from build123d import *

# Parameters (mm, degrees)
SKETCH1_W               = 8
SKETCH1_H               = 8
BOSS_EXTRUDE1_DEPTH     = 3
CUT_EXTRUDE1_DEPTH      = 12.704699911
CUT_EXTRUDE1_DEPTH_BACK = 12.704699911
CUT_EXTRUDE2_DEPTH      = 11
SKETCH4_R               = 1.75
CUT_EXTRUDE3_DEPTH      = 0.4
SKETCH5_W               = 8
SKETCH5_H               = 1
BOSS_EXTRUDE2_DEPTH     = 2
FILLET1_R               = 4
CUT_EXTRUDE4_DEPTH      = 0.4
CUT_EXTRUDE5_DEPTH      = 0.5


with BuildPart() as part:
    # Sketch1 → Boss-Extrude1 (new body)
    with BuildSketch(Plane(origin=(0, 0, 0), x_dir=(1, 0, 0), z_dir=(0, 1, 0))):
        with Locations((4, 4)):
            Rectangle(SKETCH1_W, SKETCH1_H)
    extrude(amount=BOSS_EXTRUDE1_DEPTH)

    # Sketch2 → Cut-Extrude1 (cut, two sides: drawn at the far end of the back side and taken through both)
    with BuildSketch(Plane.XY.offset(-CUT_EXTRUDE1_DEPTH_BACK)):
        Polygon((0, 0), (0.6, 3), (0, 3), align=None)
        Polygon((8, 0), (7.4, 3), (8, 3), align=None)
    extrude(amount=CUT_EXTRUDE1_DEPTH + CUT_EXTRUDE1_DEPTH_BACK, mode=Mode.SUBTRACT)

    # Sketch3 → Cut-Extrude2 (cut)
    with BuildSketch(Plane(origin=(0, 0, 0), x_dir=(0, 0, -1), z_dir=(1, 0, 0))):
        Polygon((0, 0), (0.6, 3), (0, 3), align=None)
        Polygon((8, 3), (7.4, 3), (8, 0), align=None)
    extrude(amount=CUT_EXTRUDE2_DEPTH, mode=Mode.SUBTRACT)

    # Sketch4 → Cut-Extrude3 (cut)
    with BuildSketch(Plane.XZ):
        with Locations(Location((4, -3.75, 0), (0, 0, 270))):
            Circle(SKETCH4_R)
    extrude(amount=-CUT_EXTRUDE3_DEPTH, mode=Mode.SUBTRACT)

    # Sketch5 → Boss-Extrude2 (add)
    with BuildSketch(Plane.XZ):
        with Locations((4, -7.5)):
            Rectangle(SKETCH5_W, SKETCH5_H)
    extrude(amount=BOSS_EXTRUDE2_DEPTH)

    # Fillet1
    # the kernel refuses this fillet: 4 mm, written as the material it takes off along each edge
    with BuildSketch(Plane(origin=(8, -2, -16.660254038), x_dir=(0, 1, 0), z_dir=(0, 0, 1)), Plane(origin=(0, -2, 1.660254038), x_dir=(0, 1, 0), z_dir=(0, 0, -1))) as fillet1_piece_1:
        with BuildLine():
            CenterArc((4, 3.464101615), FILLET1_R, 180, 60)
            Line((0, 3.464101615), (-0.08, 3.464101615))
            Line((-0.08, 3.464101615), (-0.08, 0))
            Line((-0.08, 0), (0, -0.08))
            ThreePointArc((0, -0.08), (1, -0.08), (1.96, -0.069282032))
            Line((1.96, -0.069282032), (2, 0))
        make_face()
    extrude(amount=18.320508076, mode=Mode.SUBTRACT)

    # Sketch6 → Cut-Extrude4 (cut)
    with BuildSketch(Plane(origin=(0, 3, 0), x_dir=(1, 0, 0), z_dir=(0, 1, 0))):
        with BuildLine():
            Line((2.413140262, 5.995145478), (3.182371031, 5.995145478))
            Line((3.182371031, 5.995145478), (3.182371031, 3.824472401))
            add(Edge.make_bspline(
                [(3.182371031, 3.824472401), (3.182664695, 3.783339968), (3.183225327, 3.704814249), (3.183611242, 3.59262518), (3.18574694, 3.491896749), (3.190378411, 3.402466647), (3.193557117, 3.32438048), (3.199459629, 3.257623918), (3.205347836, 3.202222959), (3.211072588, 3.16927001), (3.213621031, 3.154600607)],
                knots=[0, 0, 0, 0, 1.470600056, 2.807515117, 4.011048972, 5.072079398, 6.00911328, 6.804506435, 7.467811572, 8, 8, 8, 8], degree=3))
            add(Edge.make_bspline(
                [(3.213621031, 3.154600607), (3.224127628, 3.115054038), (3.244816443, 3.03718185), (3.301842427, 2.930732637), (3.377172946, 2.83690436), (3.454012852, 2.769989694), (3.523520467, 2.722632459), (3.582561491, 2.693810163), (3.645203631, 2.667536787), (3.712771176, 2.647377448), (3.784538951, 2.629737301), (3.861373833, 2.619537644), (3.942627383, 2.611709661), (3.998321517, 2.610930314), (4.026922313, 2.610530094)],
                knots=[0, 0, 0, 0, 1.376921055, 2.711331395, 4.038631339, 5.418057255, 6.132954575, 6.870556231, 7.630397752, 8.422890386, 9.247036838, 10.121396817, 11.035274583, 12, 12, 12, 12], degree=3))
            add(Edge.make_bspline(
                [(4.026922313, 2.610530094), (4.055777389, 2.611053435), (4.111957634, 2.612072369), (4.193372399, 2.618140476), (4.269330983, 2.629588903), (4.339786919, 2.644600001), (4.40511233, 2.663571514), (4.464786061, 2.687591678), (4.518714075, 2.716497769), (4.582078678, 2.760066391), (4.650258908, 2.821527538), (4.715873674, 2.905091818), (4.762833649, 2.997337694), (4.784859868, 3.081565077), (4.796180605, 3.154949811), (4.803077806, 3.219164001), (4.809385646, 3.291832182), (4.815113647, 3.372755319), (4.819030865, 3.461994153), (4.821149619, 3.559774375), (4.82281709, 3.666080391), (4.823198873, 3.739802878), (4.823396672, 3.777998042)],
                knots=[0, 0, 0, 0, 1.036876239, 2.018776863, 2.930845756, 3.794842666, 4.605604932, 5.371924355, 6.101864688, 6.799283669, 8.1310906, 9.382718023, 10.597336334, 11.822035891, 12.492591141, 13.265194674, 14.141890321, 15.11351293, 16.179860579, 17.351049011, 18.627594861, 20, 20, 20, 20], degree=3))
            Line((4.823396672, 3.777998042), (4.823396672, 5.995145478))
            Line((4.823396672, 5.995145478), (5.592627441, 5.995145478))
            Line((5.592627441, 5.995145478), (5.592627441, 3.902998042))
            add(Edge.make_bspline(
                [(5.592627441, 3.902998042), (5.592528847, 3.845305157), (5.592339402, 3.734449864), (5.589381475, 3.574956755), (5.583094941, 3.428628514), (5.577830511, 3.295214312), (5.567675642, 3.175054503), (5.557043529, 3.068074376), (5.543346947, 2.974292627), (5.523815493, 2.867696041), (5.490991615, 2.748101531), (5.438090809, 2.615994056), (5.370481989, 2.495804532), (5.288434562, 2.387071806), (5.192421188, 2.289363714), (5.081004269, 2.203064381), (4.955329501, 2.127124651), (4.84016309, 2.072443299), (4.739752735, 2.035622669), (4.65797018, 2.010704116), (4.570444093, 1.989952175), (4.477277128, 1.973483664), (4.378429252, 1.959598273), (4.273864574, 1.950325107), (4.163741291, 1.944537997), (4.088628699, 1.944091898), (4.050159493, 1.943863427)],
                knots=[0, 0, 0, 0, 1.415574045, 2.719986624, 3.913607924, 5.00929969, 5.995467356, 6.871900228, 7.64671288, 8.320227872, 9.530145585, 10.682614022, 11.803571353, 12.90325401, 14.015460715, 15.154679255, 16.351678057, 17.612271512, 18.275764165, 18.974412946, 19.708786676, 20.481351116, 21.295095879, 22.157200529, 23.056203067, 24, 24, 24, 24], degree=3))
            add(Edge.make_bspline(
                [(4.050159493, 1.943863427), (4.00394899, 1.944454117), (3.914432357, 1.945598373), (3.784491522, 1.950702797), (3.663419731, 1.961238523), (3.550836598, 1.975478544), (3.446788608, 1.993784557), (3.351012543, 2.015669281), (3.264273035, 2.043328483), (3.160959321, 2.082832512), (3.045798952, 2.143260432), (2.920442018, 2.223870786), (2.810400187, 2.314853884), (2.716640343, 2.415320705), (2.638260762, 2.521740618), (2.574552012, 2.631810814), (2.523497916, 2.743696672), (2.502164616, 2.821459533), (2.491665903, 2.859728812)],
                knots=[0, 0, 0, 0, 1.128613534, 2.186292659, 3.174878439, 4.095586888, 4.95671962, 5.754129884, 6.492676435, 7.178284149, 8.453103036, 9.659838108, 10.813193309, 11.929983019, 13.007587775, 14.033493319, 15.032227051, 16, 16, 16, 16], degree=3))
            add(Edge.make_bspline(
                [(2.491665903, 2.859728812), (2.48524032, 2.889857793), (2.471705989, 2.953319061), (2.456334745, 3.054210037), (2.442311642, 3.165307899), (2.432733679, 3.286744058), (2.423654648, 3.418133217), (2.417136225, 3.559723113), (2.414455843, 3.711481594), (2.413587623, 3.816192051), (2.413140262, 3.870145478)],
                knots=[0, 0, 0, 0, 0.728071598, 1.533551606, 2.411422299, 3.374601532, 4.412367648, 5.524718474, 6.72457895, 8, 8, 8, 8], degree=3))
            Line((2.413140262, 3.870145478), (2.413140262, 5.995145478))
        make_face()
    extrude(amount=-CUT_EXTRUDE4_DEPTH, mode=Mode.SUBTRACT)

    # Sketch7 → Cut-Extrude5 (cut)
    with BuildSketch(Plane(origin=(0, 3, 0), x_dir=(1, 0, 0), z_dir=(0, 1, 0))):
        with BuildLine():
            Line((5.850386773, 2.400368579), (5.850386773, 2.746522425))
            Line((5.850386773, 2.746522425), (7.02730985, 2.746522425))
            Line((7.02730985, 2.746522425), (7.02730985, 2.492676271))
            add(Edge.make_bspline(
                [(7.02730985, 2.492676271), (7.015032321, 2.480184286), (6.989793248, 2.454504354), (6.953640746, 2.41247659), (6.916952595, 2.366869092), (6.880495981, 2.317067299), (6.84313767, 2.263857918), (6.806519427, 2.206220957), (6.769380335, 2.144904141), (6.719379376, 2.058171383), (6.660934493, 1.944871602), (6.599102899, 1.804034186), (6.546425212, 1.658871525), (6.510353845, 1.535182236), (6.485981829, 1.436045461), (6.470058334, 1.363554301), (6.45665413, 1.293103137), (6.44574982, 1.224568153), (6.437611625, 1.157918082), (6.431181064, 1.093384645), (6.428008496, 1.030810475), (6.427540351, 0.989794441), (6.42730985, 0.969599348)],
                knots=[0, 0, 0, 0, 0.628545797, 1.29210959, 1.98878689, 2.729126096, 3.507039704, 4.322017351, 5.179550397, 6.080149501, 7.915136253, 9.752312618, 11.597470118, 13.454141581, 14.373891568, 15.261584755, 16.117868869, 16.947726723, 17.752002974, 18.527724242, 19.275094557, 20, 20, 20, 20], degree=3))
            Line((6.42730985, 0.969599348), (6.081156004, 0.969599348))
            add(Edge.make_bspline(
                [(6.081156004, 0.969599348), (6.082313464, 1.000264514), (6.084641243, 1.061935513), (6.093350513, 1.15450167), (6.107029358, 1.247412503), (6.124019401, 1.340882746), (6.146450494, 1.434684851), (6.172051243, 1.529166286), (6.203062702, 1.623822431), (6.237825714, 1.718472296), (6.276202253, 1.812217257), (6.31802728, 1.903894573), (6.363192674, 1.992932291), (6.411111069, 2.079643245), (6.462339924, 2.16374848), (6.516917811, 2.245156666), (6.574070556, 2.324456683), (6.614935451, 2.375068877), (6.635362734, 2.400368579)],
                knots=[0, 0, 0, 0, 0.943249748, 1.896978291, 2.856365892, 3.829648507, 4.816416106, 5.820376826, 6.838120354, 7.877341886, 8.919613352, 9.951365796, 10.974227495, 11.988073359, 12.996274698, 14.000568529, 15.000536908, 16, 16, 16, 16], degree=3))
            Line((6.635362734, 2.400368579), (5.850386773, 2.400368579))
        make_face()
    extrude(amount=-CUT_EXTRUDE5_DEPTH, mode=Mode.SUBTRACT)


solid = part.part
Geometry: final body of the model. Coordinates: model frame, mm. A direction names the side the tool comes from. Coordinates: 2 decimals unless noted, no trailing zeros. Write each loop counter-clockwise with the first axis right and the second up, starting at its lowest first coordinate (ties: lowest second). Pieces come first, ordered by that corner, then holes. Notation, with made-up numbers: (36, 0) - (45, 0) arc R21 ccw to (45, 37) - close; hole circle Ø7 at (-28.75, 49.5). An arc over 180 degrees is marked (long way). Return JSON: item names as keys, results as strings.
Item 1: Line query: L1, parallel to Y at x = 1.75, z = -4.5; L2, parallel to X at y = 0.3, z = -3.75; L3, parallel to X at y = 0.1, z = -3.75. Output: solid intervals per line, ascending.
Completed:
{"L1": "y = 0 to 3", "L2": "x = 0.06 to 2.25, 5.75 to 7.94", "L3": "x = 0.02 to 2.25, 5.75 to 7.98"}
Item 2: Pull-direction query (Z, two-part tool) for faces 1 (the face through (4, 0.4, -4)), 2 (the face through (3.9, 1.5, -7.7)), 3 (the face through (4, -1, -7)); classes: +Z half, -Z half, draft (parallel to the pull), parting line (faces both ways), or undercut.
Completed:
{"face 1": "undercut", "face 2": "-Z half", "face 3": "+Z half"}
Item 3: Section query C-C (y = 1.15). Output: boundary loops of the cut face in (x, z), and give its area (3 significant figures).
Completed:
{"outline": "(0.23, -7.77) - (7.77, -7.77) - (7.77, -0.23) - (0.23, -0.23) - close", "area": "56.9 mm2"}
Item 4: Reachability of faces 4 (the face through (4, -2, -7.5)), 5 (the face through (3, 2.6, -4)), 6 (the face through (3, 0, -2)), 7 (the face through (2.94, 0.2, -2.36)) from +Z, -Z, +X, -X, +Y, -Y: full face, straight path, thin tool, end or side. Return the list, or none.
Completed:
{"face 4": "+Z, -Z, +X, -X, -Y", "face 5": "+Y", "face 6": "+Z, +X, -X, -Y", "face 7": "-Y"}
Item 5: Pin query (flat end, axial travel): pin 1 Ø2 at (y, z) = (1.5, -4.5) entering from +X; pin 2 Ø1.8 at (x, z) = (4.5, -4) entering from -Y; pin 3 Ø4 at (x, z) = (6, -3.5) entering from -Y. Return the tip coordinate at first contact, or that it passes through.
Completed:
{"pin 1": "stops at x = 7.9", "pin 2": "stops at y = 0.4", "pin 3": "stops at y = 0"}
Item 6: Section query A-A (y = 0.3). Output: boundary loops of the cut face in (x, z), and give its area (3 significant figures).
Completed:
{"outline": "(0.06, -7.94) - (7.94, -7.94) - (7.94, -0.06) - (0.06, -0.06) - close; hole circle Ø3.5 at (4, -3.75)", "area": "52.5 mm2"}
Item 7: Section query B-B (z = -7.25). Output: boundary loops of the cut face in (x, y).
Completed:
{"outline": "(0, 0) arc R4 ccw to (3.46, -2) - (4.54, -2) arc R4 ccw to (8, 0) - (7.4, 3) - (0.6, 3) - close"}
Item 8: Section query D-D (y = -1.45). Output: boundary loops of the cut face in (x, z).
Completed:
{"outline": "(1.44, -8) - (6.56, -8) - (6.56, -7) - (1.44, -7) - close"}
